Answer from the drawing. Dimensions are ordinates in mm from the lowest x, y and z of the part. Round coordinates to 2 decimals unless told otherwise and drop trailing zeros. Loops run counter-clockwise (first coordinate to the right, second up) from the corner with the lowest first, then second, coordinate; pieces in that order, holes last. Notation, with made-up numbers: (-12, -29) - (33, -29) arc R16 ccw to (33, -19) - close; hole circle Ø1 at (5, 26). An arc over 180 degrees is marked (long way). Answer as CSV lines item,"result". Start each with the question number.
Q1. Section D-D on x = 99.5 is taken. Write down the section's boundary in (y, z).
Q2. Each of these flat-tipped pins is pushed along its axis until it touches: pin 1 Ø11.5 at (x, y) = (60, 40) entering from -Z; pin 2 Ø1 at (x, z) = (39, 3.5) entering from -Y. Where does it stop, or does it pass through?
Q3. Straight lines are drawn through the part: L1, parallel to Y at x = 96, z = 0.6; L2, parallel to Y at x = 75.5, z = 3.35. For each, find the intervals that lie inside material, in ascending order. Write a range as [from, to].
Q4. Section C-C on y = 40 is taken. Write down the section's boundary in (x, z), then the cut area to 3 significant figures.
Q5. Section B-B on x = 60 is taken. Write down the section's boundary in (y, z).
Q6. Section A-A on z = 2.25 is taken. Write down the section's boundary in (x, y), then the cut area to 3 significant figures.
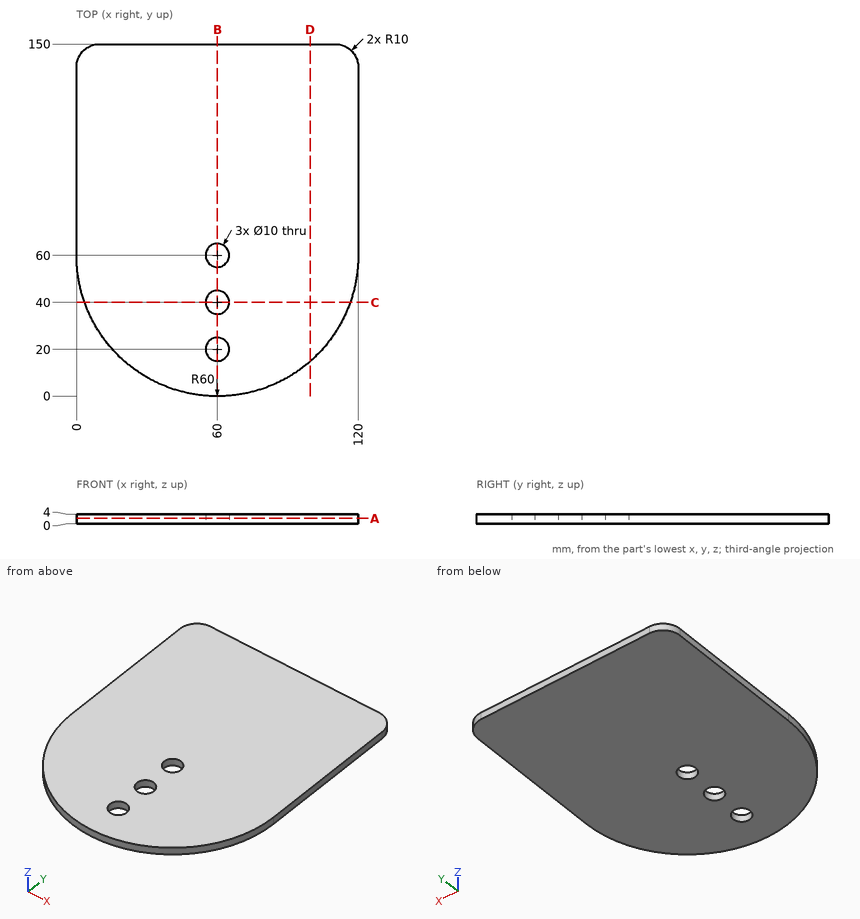
Findings:
1,outline,"(14.84, 0) - (150, 0) - (150, 4) - (14.84, 4) - close"
2,pin 1,"stops at z = 0"
2,pin 2,"stops at y = 3.61"
3,L1,"y = [12, 150]"
3,L2,"y = [2.04, 150]"
4,outline,"(3.43, 0) - (55, 0) - (55, 4) - (3.43, 4) - close; (65, 0) - (116.57, 0) - (116.57, 4) - (65, 4) - close"
4,area,"413 mm^2"
5,outline,"(0, 0) - (15, 0) - (15, 4) - (0, 4) - close; (25, 0) - (35, 0) - (35, 4) - (25, 4) - close; (45, 0) - (55, 0) - (55, 4) - (45, 4) - close; (65, 0) - (150, 0) - (150, 4) - (65, 4) - close"
6,outline,"(0, 60) arc R60 ccw to (120, 60) - (120, 140) arc R10 ccw to (110, 150) - (10, 150) arc R10 ccw to (0, 140) - close; hole circle Ø10 at (60, 20); hole circle Ø10 at (60, 40); hole circle Ø10 at (60, 60)"
6,area,"16,200 mm^2"
